Check sheet for the modelled part. Datum: model origin and axes. Units: mm. Face numbers are marked on the shaded views. Give positions to 0.01 mm unless a question says otherwise; leave off trailing zeros. Write each loop counter-clockwise with the first axis right and the second up, starting at its lowest first coordinate (ties: lowest second). Pieces come first, ordered by that corner, then holes. Notation, with made-up numbers: (83, 79.5) -> (137, 79.5) arc R17 ccw to (137, 92.5) -> close; hole circle Ø11 at (36.25, 7.25). An arc over 180 degrees is marked (long way). Use a Markdown table: item, result. Add a question column.
1. Cross-section at C-C (z = 10). Enter the section's corners in (x, y).
2. Cross-section at A-A (x = 10.5). Enter the section's corners in (y, z).
3. Release check for a two-part mould opening along Y. For the marked faces 1, 2 and 3 record: released by +Y, released by -Y, zero draft, split by the parting line, or undercut.
4. Gauge pin test, flat ends, axial feed: P1, Ø3, axis at x = 23.5, y = 18.5, coming from the +Z side; P2, Ø6, axis at x = 14, z = 2.5, coming from the +Y side; P3, Ø4.5, axis at x = -7.5, z = 7.5, coming from the -Y side; P4, Ø1.5, axis at y = 1.5, z = 5, coming from the +X side. Record the tip position at first contact, or that the pin passes through.
5. Cross-section at D-D (y = -1.75). Enter the section's corners in (x, z), then the cut area to 3 significant figures.
6. Scan lines: probe 1 along Z at (x, y) = (-7, 0); probe 2 along Y at (x, z) = (24.5, 7); probe 3 along Y at (x, z) = (15, 17). Record each from-to range of solid material in increasing order. Write a range as [from, to].
7. Cross-section at B-B (z = 2.75). Enter the section's corners in (x, y), then the cut area to 3 significant figures.
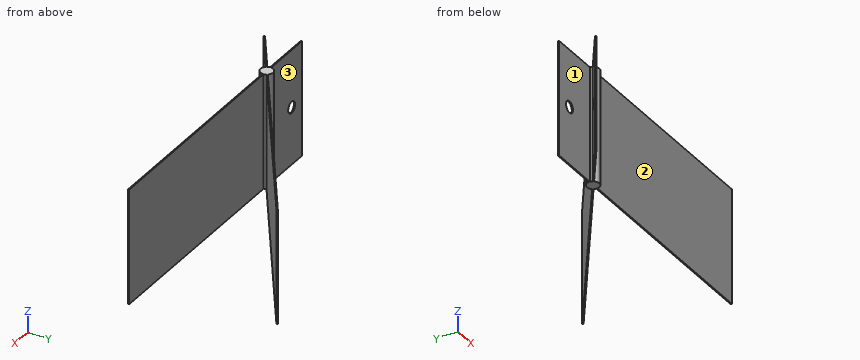
from build123d import *

# Parameters (mm, degrees)
EXTRUDE_1_DEPTH          = 20
CUT_EXTRUDE_1_DEPTH      = 20
CUT_EXTRUDE_1_DEPTH_BACK = 1
CUT_EXTRUDE_2_DEPTH      = 1


with BuildPart() as part:
    # 草图1 → 凸台-拉伸1 (new body)
    with BuildSketch(Plane.XY):
        with BuildLine():
            Line((1.095445115, 0.1), (40, 0.1))
            Line((40, 0.1), (40, -0.1))
            Line((40, -0.1), (1.095445115, -0.1))
            ThreePointArc((1.095445115, -0.1), (0.314917655, -1.053957718), (-0.861015843, -0.684581418))
            Line((-0.861015843, -0.684581418), (-8.30591358, -5.569721681))
            Line((-8.30591358, -5.569721681), (-8.415635859, -5.402506186))
            Line((-8.415635859, -5.402506186), (-0.970738122, -0.517365924))
            ThreePointArc((-0.970738122, -0.517365924), (-1.053957718, -0.314917655), (-1.095445115, -0.1))
            Line((-1.095445115, -0.1), (-10, -0.1))
            Line((-10, -0.1), (-10, 0.1))
            Line((-10, 0.1), (-1.095445115, 0.1))
            ThreePointArc((-1.095445115, 0.1), (-0.314917655, 1.053957718), (0.861015843, 0.684581418))
            Line((0.861015843, 0.684581418), (33.388237738, 22.028063482))
            Line((33.388237738, 22.028063482), (33.497960016, 21.860847988))
            Line((33.497960016, 21.860847988), (0.970738122, 0.517365924))
            ThreePointArc((0.970738122, 0.517365924), (1.053957718, 0.314917655), (1.095445115, 0.1))
        make_face()
    extrude(amount=EXTRUDE_1_DEPTH)

    # 草图2 → 切除-拉伸1 (cut, two sides)
    with BuildSketch(Plane(origin=(0, 0.1, 0), x_dir=(1, 0, 0), z_dir=(0, 1, 0))) as cut_extrude_1_sk:
        with BuildLine():
            ThreePointArc((-6, -10), (-7, -9), (-8, -10))
            Line((-8, -10), (-6, -10))
        make_face()
        with BuildLine():
            Line((-6, -10), (-8, -10))
            ThreePointArc((-8, -10), (-7, -11), (-6, -10))
        make_face()
    extrude(amount=CUT_EXTRUDE_1_DEPTH, mode=Mode.SUBTRACT)
    extrude(cut_extrude_1_sk.sketch, amount=-CUT_EXTRUDE_1_DEPTH_BACK, mode=Mode.SUBTRACT)

    # 草图3 → 切除-拉伸2 (cut)
    with BuildSketch(Plane(origin=(0.054861139, -0.083607747, 0), x_dir=(0.836077472, 0.548611393, 0), z_dir=(0.548611393, -0.836077472, 0))):
        with BuildLine():
            ThreePointArc((-6, 10), (-7, 11), (-8, 10))
            Line((-8, 10), (-6, 10))
        make_face()
        with BuildLine():
            Line((-6, 10), (-8, 10))
            ThreePointArc((-8, 10), (-7, 9), (-6, 10))
        make_face()
    extrude(amount=-CUT_EXTRUDE_2_DEPTH, mode=Mode.SUBTRACT)


solid = part.part
Worked answers:
| question | item | result |
|---|---|---|
| 1 | outline | (-10, -0.1) -> (-8, -0.1) -> (-8, 0.1) -> (-10, 0.1) -> close; (-8.42, -5.4) -> (-8.31, -5.57) -> (-6.63, -4.47) -> (-6.74, -4.31) -> close; (-6, -0.1) -> (-1.1, -0.1) arc R1.1 ccw to (-0.97, -0.52) -> (-5.07, -3.21) -> (-4.96, -3.38) -> (-0.86, -0.68) arc R1.1 ccw to (1.1, -0.1) -> (40, -0.1) -> (40, 0.1) -> (1.1, 0.1) arc R1.1 ccw to (0.97, 0.52) -> (33.5, 21.86) -> (33.39, 22.03) -> (0.86, 0.68) arc R1.1 ccw to (-1.1, 0.1) -> (-6, 0.1) -> close |
| 2 | outline | (-0.1, 0) -> (0.1, 0) -> (0.1, 20) -> (-0.1, 20) -> close; (6.77, 0) -> (7.01, 0) -> (7.01, 20) -> (6.77, 20) -> close |
| 3 | face 1 | undercut |
| 3 | face 2 | released by -Y |
| 3 | face 3 | released by +Y |
| 4 | P1 | passes through |
| 4 | P2 | stops at y = 11.27 |
| 4 | P3 | stops at y = -5.57 |
| 4 | P4 | stops at x = 3.61 |
| 5 | outline | (-2.85, 0) -> (-2.48, 0) -> (-2.48, 20) -> (-2.85, 20) -> close |
| 5 | area | 7.29 mm² |
| 6 | probe 1 | z = [0, 9], [11, 20] |
| 6 | probe 2 | y = [-0.1, 0.1], [15.96, 16.2] |
| 6 | probe 3 | y = [-0.1, 0.1], [9.72, 9.96] |
| 7 | outline | (-10, -0.1) -> (-1.1, -0.1) arc R1.1 ccw to (-0.97, -0.52) -> (-8.42, -5.4) -> (-8.31, -5.57) -> (-0.86, -0.68) arc R1.1 ccw to (1.1, -0.1) -> (40, -0.1) -> (40, 0.1) -> (1.1, 0.1) arc R1.1 ccw to (0.97, 0.52) -> (33.5, 21.86) -> (33.39, 22.03) -> (0.86, 0.68) arc R1.1 ccw to (-1.1, 0.1) -> (-10, 0.1) -> close |
| 7 | area | 22.9 mm² |
